Verification items for the finished model (mm, model axes). Face numbers are marked on the shaded views. A direction names the side the tool comes from. Coordinates: 2 decimals unless noted, no trailing zeros. Order: outer loops, then holes, each group sorted by start corner. A loop starts at its lowest first (then second) coordinate and runs counter-clockwise, first axis right, second up. Notation, with made-up numbers: M -21,-3 L 7,-3 A38 ccw 7,36 Z; hole C 61.25,30.5 d9. An arc over 180 degrees is marked long. Return JSON: item names as keys, results as strings. Group by question number.
Q1. Go/stop test with flat-tipped pins: pin 1 Ø3 at (x, y) = (0, 9.5) entering from +Z; pin 2 Ø1.6 at (x, y) = (0, 50.5) entering from +Z; pin 3 Ø4 at (x, z) = (22.5, 11.25) entering from +Y; pin 4 Ø7.5 at (x, y) = (-1, 39) entering from -Z. Record where each tip stops, or that it passes through.
Q2. Section check C-C, the plane z = 1. Enter the section's corners in (x, y).
Q3. Mould release check, pull along Z, two halves, no side actions. Record for the marked faces 1, 2, 3 and 4: pulls with the +Z half, pulls with the -Z half, needs draft (parallel to the pull), parting line crosses it, or undercut.
Q4. Access from +Z, -Z, +X, -X, +Y, -Y to the whole of each face (thin tool, end or side, straight path). Record for the marked faces 5, 6, 7, 8 and 9.
Q5. Section check D-D, the plane x = 13. Enter the section's corners in (y, z).
Q6. Thickness scan on probe 1 along Y at (x, z) = (0, 13.05); probe 2 along Y at (x, z) = (13, -13); probe 3 along Z at (x, y) = (-19, 5.5). Record the ranges inside material, lowest first.
Q7. Section check A-A, the plane x = 0. Count the separate pieces of the cut face and the enclosed holes in it, then the cut area to 3 significant figures.
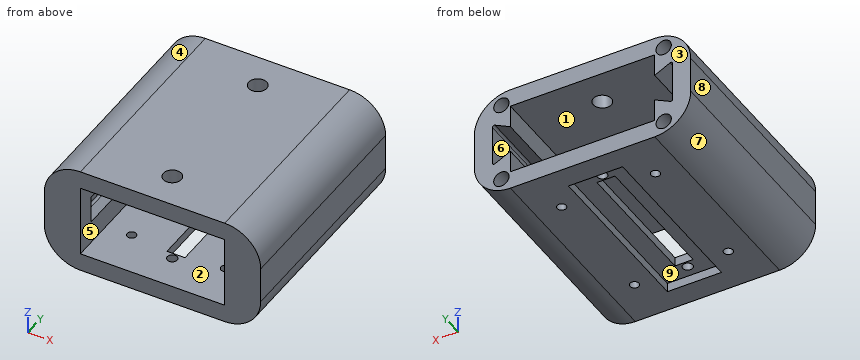
from build123d import *

# Parameters (mm, degrees)
SKETCH1_W           = 60
SKETCH1_H           = 30
SKETCH1_W_2         = 40
SKETCH1_H_2         = 20
BOSS_EXTRUDE1_DEPTH = 5
SKETCH2_W           = 60
SKETCH2_H           = 30
BOSS_EXTRUDE2_DEPTH = 55
SKETCH4_R           = 1.375
SKETCH4_W           = 5
SKETCH4_H           = 37.5
CUT_EXTRUDE1_DEPTH  = 5
SKETCH5_W           = 15
SKETCH5_H           = 47.5
CUT_EXTRUDE2_DEPTH  = 2.5
FILLET1_R           = 10
SKETCH6_R           = 2.125
CUT_EXTRUDE3_DEPTH  = 5
SKETCH7_R           = 2.5
CUT_EXTRUDE4_DEPTH  = 5
SKETCH8_R           = 1.25
CUT_EXTRUDE5_DEPTH  = 5


with BuildPart() as part:
    # Sketch1 → Boss-Extrude1 (new body)
    with BuildSketch(Plane(origin=(0, 0, 0), x_dir=(1, 0, 0), z_dir=(0, 1, 0))):
        Rectangle(SKETCH1_W, SKETCH1_H)
        Rectangle(SKETCH1_W_2, SKETCH1_H_2, mode=Mode.SUBTRACT)
    extrude(amount=BOSS_EXTRUDE1_DEPTH)

    # Sketch2 → Boss-Extrude2 (add)
    with BuildSketch(Plane(origin=(0, 5, 0), x_dir=(1, 0, 0), z_dir=(0, 1, 0))):
        Rectangle(SKETCH2_W, SKETCH2_H)
        with BuildLine():
            Line((20, 10), (20, 3.75))
            Line((20, 3.75), (24.276393202, 5.888196601))
            ThreePointArc((24.276393202, 5.888196601), (24.762865556, 5.86630841), (25, 5.440983006))
            Line((25, 5.440983006), (25, -5.440983006))
            ThreePointArc((25, -5.440983006), (24.762865556, -5.86630841), (24.276393202, -5.888196601))
            Line((24.276393202, -5.888196601), (20, -3.75))
            Line((20, -3.75), (20, -10))
            Line((20, -10), (-20, -10))
            Line((-20, -10), (-20, -3.75))
            Line((-20, -3.75), (-24.276393202, -5.888196601))
            ThreePointArc((-24.276393202, -5.888196601), (-24.762865556, -5.86630841), (-25, -5.440983006))
            Line((-25, -5.440983006), (-25, 5.440983006))
            ThreePointArc((-25, 5.440983006), (-24.762865556, 5.86630841), (-24.276393202, 5.888196601))
            Line((-24.276393202, 5.888196601), (-20, 3.75))
            Line((-20, 3.75), (-20, 10))
            Line((-20, 10), (20, 10))
        make_face(mode=Mode.SUBTRACT)
    extrude(amount=BOSS_EXTRUDE2_DEPTH)

    # Sketch4 → Cut-Extrude1 (cut)
    with BuildSketch(Plane(origin=(-36.213203436, 0, -15), x_dir=(1, 0, 0), z_dir=(0, 0, 1))):
        with Locations(Location((36.213203436, 50.5, 0), (0, 0, 180))):
            Circle(SKETCH4_R)
        with Locations(Location((36.213203436, 9.5, 0), (0, 0, 180))):
            Circle(SKETCH4_R)
        with Locations((36.213203436, 30)):
            Rectangle(SKETCH4_W, SKETCH4_H)
    extrude(amount=CUT_EXTRUDE1_DEPTH, mode=Mode.SUBTRACT)

    # Sketch5 → Cut-Extrude2 (cut)
    with BuildSketch(Plane(origin=(0, 0, -15), x_dir=(-1, 0, 0), z_dir=(0, 0, -1))):
        with Locations((0, 30)):
            Rectangle(SKETCH5_W, SKETCH5_H)
    extrude(amount=-CUT_EXTRUDE2_DEPTH, mode=Mode.SUBTRACT)

    # Fillet1
    fillet1_edges = [part.edges().sort_by_distance(p)[0] for p in [
        (30, 30, 15),
        (-30, 30, 15),
        (-30, 30, -15),
        (30, 30, -15),
    ]]
    fillet(fillet1_edges, radius=FILLET1_R)

    # Sketch6 → Cut-Extrude3 (cut)
    with BuildSketch(Plane(origin=(0, 60, 0), x_dir=(1, 0, 0), z_dir=(0, 1, 0))):
        with Locations(Location((-22.5, 11.25, 0), (0, 0, 270))):
            Circle(SKETCH6_R)
        with Locations(Location((22.5, 11.25, 0), (0, 0, 270))):
            Circle(SKETCH6_R)
        with Locations(Location((-22.5, -11.25, 0), (0, 0, 270))):
            Circle(SKETCH6_R)
        with Locations(Location((22.5, -11.25, 0), (0, 0, 270))):
            Circle(SKETCH6_R)
    extrude(amount=-CUT_EXTRUDE3_DEPTH, mode=Mode.SUBTRACT)

    # Sketch7 → Cut-Extrude4 (cut)
    with BuildSketch(Plane.XY.offset(15)):
        with Locations((0, 50.5)):
            Circle(SKETCH7_R)
        with Locations((0, 9.5)):
            Circle(SKETCH7_R)
    extrude(amount=-CUT_EXTRUDE4_DEPTH, mode=Mode.SUBTRACT)

    # Sketch8 → Cut-Extrude5 (cut)
    with BuildSketch(Plane(origin=(0, 0, -15), x_dir=(-1, 0, 0), z_dir=(0, 0, -1))):
        with Locations((-13, 47.5)):
            Circle(SKETCH8_R)
        with Locations((13, 47.5)):
            Circle(SKETCH8_R)
        with Locations((-13, 12.5)):
            Circle(SKETCH8_R)
        with Locations((13, 12.5)):
            Circle(SKETCH8_R)
    extrude(amount=-CUT_EXTRUDE5_DEPTH, mode=Mode.SUBTRACT)


solid = part.part
Numbers:
{
 "1": {"pin 1": "stops at z = -10", "pin 2": "passes through", "pin 3": "stops at y = 55", "pin 4": "stops at z = -12.5"},
 "2": {"outline": "M -30,0 L -20,0 L -20,5 L -25,5 L -25,60 L -30,60 Z; M 20,0 L 30,0 L 30,60 L 25,60 L 25,5 L 20,5 Z"},
 "3": {"face 1": "undercut", "face 2": "undercut", "face 3": "needs draft", "face 4": "pulls with the +Z half"},
 "4": {"face 5": "+Y, -Y", "face 6": "+Y", "face 7": "-Z, -X, +Y, -Y", "face 8": "+Z, -Z, -X, +Y, -Y", "face 9": "-Z"},
 "5": {"outline": "M 0,-15 L 11.25,-15 L 11.25,-10 L 0,-10 Z; M 0,10 L 60,10 L 60,15 L 0,15 Z; M 13.75,-15 L 46.25,-15 L 46.25,-10 L 13.75,-10 Z; M 48.75,-15 L 60,-15 L 60,-10 L 48.75,-10 Z"},
 "6": {"probe 1": "y = 0 to 7, 12 to 48, 53 to 60", "probe 2": "y = 0 to 11.25, 13.75 to 46.25, 48.75 to 60", "probe 3": "z = -15 to -10, 10 to 15"},
 "7": {"separate pieces": "7", "enclosed holes": "0", "area": "324 mm2"}
}
